Model file for the job. Use its own axes, mm. Coordinates: 2 decimals unless noted, no trailing zeros. Order: outer loops, then holes, each group sorted by start corner. A loop starts at its lowest first (then second) coordinate and runs counter-clockwise, first axis right, second up.
from build123d import *

# Parameters (mm, degrees)
SKETCH_55_W         = 87
SKETCH_55_H         = 42
EXTRUDE_1_DEPTH     = 1.6
SKETCH_56_W         = 13
SKETCH_56_H         = 16.6
CUT_EXTRUDE_1_DEPTH = 1.6
FILLET_1_R          = 0.5


with BuildPart() as part:
    # Эскиз55 → Бобышка-Вытянуть1 (new body)
    with BuildSketch(Plane(origin=(0, 0, 0), x_dir=(1, 0, 0), z_dir=(0, 1, 0))):
        with Locations((43.5, 21)):
            Rectangle(SKETCH_55_W, SKETCH_55_H)
    extrude(amount=EXTRUDE_1_DEPTH)

    # Эскиз56 → Вырез-Вытянуть1 (cut)
    with BuildSketch(Plane(origin=(0, 1.6, 0), x_dir=(1, 0, 0), z_dir=(0, 1, 0))):
        with Locations((80.5, 33.7)):
            Rectangle(SKETCH_56_W, SKETCH_56_H)
    extrude(amount=-CUT_EXTRUDE_1_DEPTH, mode=Mode.SUBTRACT)

    # Скругление1
    fillet_1_edges = [part.edges().sort_by_distance(p)[0] for p in [
        (87, 1.6, -12.7),
        (37, 1.6, -42),
        (74, 0.8, -25.4),
        (74, 1.6, -33.7),
        (80.5, 1.6, -25.4),
        (0, 1.6, -21),
        (43.5, 1.6, 0),
    ]]
    fillet(fillet_1_edges, radius=FILLET_1_R)


solid = part.part
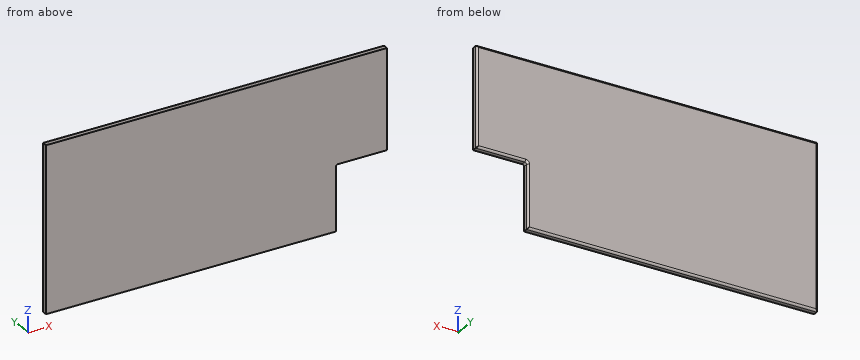
Q1. Probe line 1 (X direction, y = 1.2, z = -17.5); line 2 (Z direction, x = 30, y = 1.2); line 3 (X direction, y = 0.85, z = -39.5). List the from-to ranges inside material, lowest first.
Established:
line 1: x = 0.01 to 86.99
line 2: z = -41.99 to -0.01
line 3: x = 0 to 74
Q2. Cut at C-C, the plane x = 81.5. List the corners of the cut face in (y, z), plus the area to 3 significant figures.
Established:
outline: (0, -25.4) - (1.1, -25.4) arc R0.5 ccw to (1.6, -24.9) - (1.6, -0.5) arc R0.5 ccw to (1.1, 0) - (0, 0) - close
area: 40.5 mm2
Q3. Drop flat-ended pins along their axis: P1, Ø0.9, axis at x = 79, y = 0.5, coming from the -Z side; P2, Ø0.9, axis at y = 0.5, z = -36.5, coming from the +X side. Give the stop position or say it passes through.
Established:
P1: stops at z = -25.4
P2: stops at x = 74
Q4. Cut at B-B, the plane z = -39. List the corners of the cut face in (x, y), plus the area to 3 significant figures.
Established:
outline: (0, 0) - (74, 0) - (74, 1.1) arc R0.5 ccw to (73.5, 1.6) - (0.5, 1.6) arc R0.5 ccw to (0, 1.1) - close
area: 118 mm2
Q5. Cut at A-A, the plane y = 0.4. List the corners of the cut face in (x, z).
Established:
outline: (0, -42) - (74, -42) - (74, -25.9) arc R0.5 cw to (74.5, -25.4) - (87, -25.4) - (87, 0) - (0, 0) - close
